Source: CAD feature listing. Evaluate the final solid. Frame: model axes, mm. Give positions to 0.01 mm unless a question says otherwise; leave off trailing zeros. Write each loop counter-clockwise with the first axis right and the second up, starting at its lowest first coordinate (ties: lowest second). Pieces come first, ordered by that corner, then holes. Notation, with made-up numbers: (80.5, 40) - (105.5, 40) arc R18 ccw to (105.5, 48) - close; hole circle Ø8 at (22, -3). An arc over 180 degrees is marked (long way). One line per question, with ' | ' between items. Start each with the question number.
(1) Pin query (flat end, axial travel): pin 1 (1.5 mm diameter, centred on x = 23.5, z = 2, fed in from +Y); pin 2 (2.5 mm diameter, centred on x = 108.5, z = 2.5, fed in from +Y); pin 3 (2.5 mm diameter, centred on x = 21.5, z = 2, fed in from +Y); pin 4 (5 mm diameter, centred on x = 63.5, y = 86.5, fed in from -Z). Return the tip coordinate at first contact, or that it passes through.
(2) Section A-A, the plane x = 101.6. Return loops of the section in (y, z), plus the area to 3 significant figures.
(3) Ray query, line 1 (Y direction, x = 101.6, z = 3.3); line 2 (X direction, y = 212, z = 0.3); line 3 (X direction, y = 135, z = 4.5). Return the intervals inside material, ascending. Write a range as [from, to].
(4) Section B-B, the plane y = 36. State how many separate pieces and enclosed holes the cut face has, plus the area to 3 significant figures.
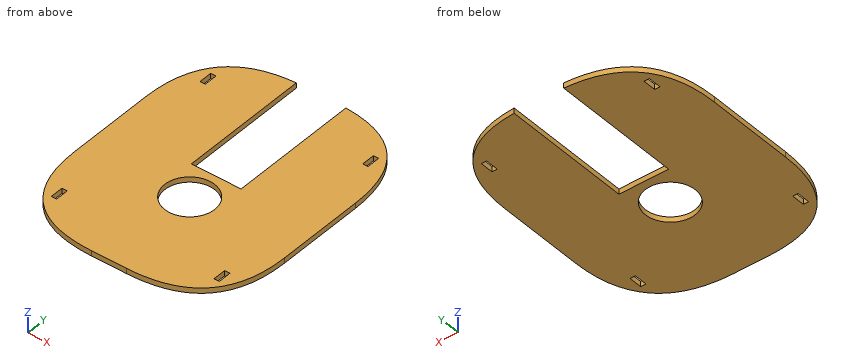
```python
from build123d import *

# Parameters (mm, degrees)
SKETCH1_W           = 203.2
SKETCH1_H           = 254
BOSS_EXTRUDE1_DEPTH = 5.08
FILLET1_SIZE        = 84.666666667
SKETCH2_R           = 24.13
CUT_EXTRUDE1_DEPTH  = 326.318377121
SKETCH8_W           = 48.006
SKETCH8_H           = 125.503270334
CUT_EXTRUDE6_DEPTH  = 326.318377121
CUT_EXTRUDE7_DEPTH  = 326.198087964


with BuildPart() as part:
    # Sketch1 → Boss-Extrude1 (new body)
    with BuildSketch(Plane.XY):
        with Locations((101.6, 127)):
            Rectangle(SKETCH1_W, SKETCH1_H)
    extrude(amount=BOSS_EXTRUDE1_DEPTH)

    # Fillet1
    # a fillet whose section is not a circle: 84.666666667 mm, written as the material it takes off along each edge
    with BuildSketch(Plane(origin=(203.2, 254, -211.666666667), x_dir=(0, -1, 0), z_dir=(0, 0, 1)), Plane(origin=(0, 254, -211.666666667), x_dir=(1, 0, 0), z_dir=(0, 0, 1)), Plane(origin=(203.2, 0, -211.666666667), x_dir=(-1, 0, 0), z_dir=(0, 0, 1))) as fillet1_piece_1:
        with BuildLine():
            Bezier((FILLET1_SIZE, 0), (0, 0), (0, -FILLET1_SIZE), weights=[1, 1, 1])
            Line((0, -FILLET1_SIZE), (0, 0))
            Line((0, 0), (FILLET1_SIZE, 0))
        make_face()
    extrude(amount=428.413333333, mode=Mode.SUBTRACT)
    with BuildSketch(Plane(origin=(0, 0, -211.666666667), x_dir=(1, 0, 0), z_dir=(0, 0, 1))) as fillet1_piece_2:
        with BuildLine():
            Bezier((FILLET1_SIZE, 0), (0, 0), (0, FILLET1_SIZE), weights=[1, 1, 1])
            Line((0, FILLET1_SIZE), (0, 0))
            Line((0, 0), (FILLET1_SIZE, 0))
        make_face()
    extrude(amount=428.413333333, mode=Mode.SUBTRACT)

    # Sketch2 → Cut-Extrude1 (cut, through all)
    with BuildSketch(Plane.XY.offset(5.08)):
        with Locations((101.6, 96.746729666)):
            Circle(SKETCH2_R)
    extrude(amount=-CUT_EXTRUDE1_DEPTH, mode=Mode.SUBTRACT)

    # Sketch8 → Cut-Extrude6 (cut, through all)
    with BuildSketch(Plane.XY.offset(5.08)):
        with Locations((101.6, 191.248364833)):
            Rectangle(SKETCH8_W, SKETCH8_H)
    extrude(amount=-CUT_EXTRUDE6_DEPTH, mode=Mode.SUBTRACT)

    # Sketch7 → Cut-Extrude7 (cut, through all)
    with BuildSketch(Plane.XY.offset(5.08)):
        Polygon((25.4, 215.9), (25.4, 222.25), (20.32, 222.25), (20.32, 209.55), (25.4, 209.55), align=None)
        Polygon((177.8, 215.9), (177.8, 222.25), (182.88, 222.25), (182.88, 209.55), (177.8, 209.55), align=None)
        Polygon((177.8, 38.1), (177.8, 44.45), (182.88, 44.45), (182.88, 31.75), (177.8, 31.75), align=None)
        Polygon((25.4, 38.1), (25.4, 44.45), (20.32, 44.45), (20.32, 31.75), (25.4, 31.75), align=None)
    extrude(amount=-CUT_EXTRUDE7_DEPTH, mode=Mode.SUBTRACT)


solid = part.part
```
Check sheet entries:
1) pin 1: y = 235.71 | pin 2: y = 128.5 | pin 3: y = 234.36 | pin 4: z = 0
2) outline: (0, 0) - (72.62, 0) - (72.62, 5.08) - (0, 5.08) - close; (120.88, 0) - (128.5, 0) - (128.5, 5.08) - (120.88, 5.08) - close | area: 408 mm²
3) line 1: [0, 72.62], [120.88, 128.5] | line 2: [7.4, 20.32], [25.4, 77.6], [125.6, 177.8], [182.88, 195.8] | line 3: [0, 77.6], [125.6, 203.2]
4) separate pieces: 3 | enclosed holes: 0 | area: 877 mm²
